from build123d import *

# Parameters (mm, degrees)
SKETCH1_R           = 3.525
SKETCH1_R_2         = 3.53
SKETCH1_R_3         = 3.535
SKETCH1_R_4         = 3.54
SKETCH1_R_5         = 3.545
SKETCH1_R_6         = 3.555
SKETCH1_R_7         = 3.56
SKETCH1_R_8         = 3.565
SKETCH1_R_9         = 3.57
SKETCH1_R_10        = 3.58
SKETCH1_R_11        = 3.585
SKETCH1_R_12        = 3.59
SKETCH1_R_13        = 3.595
SKETCH1_R_14        = 3.605
SKETCH1_R_15        = 3.615
SKETCH1_R_16        = 3.55
SKETCH1_R_17        = 3.575
SKETCH1_R_18        = 3.6
BOSS_EXTRUDE1_DEPTH = 7.62


with BuildPart() as part:
    # Sketch1 → Boss-Extrude1 (new body)
    with BuildSketch(Plane(origin=(0, 0, 0), x_dir=(1, 0, 0), z_dir=(0, 1, 0))):
        Polygon((0, 0), (43.396152207, 0), (43.396152207, 27.288237387), (26.088694952, 27.288237387), (26.088694952, 35.171413764), (0, 35.171413764), align=None)
        with Locations((4.997445859, 4.997445859)):
            Circle(SKETCH1_R, mode=Mode.SUBTRACT)
        with Locations((13.379445859, 4.997445859)):
            Circle(SKETCH1_R_2, mode=Mode.SUBTRACT)
        with Locations((21.761445859, 4.997445859)):
            Circle(SKETCH1_R_3, mode=Mode.SUBTRACT)
        with Locations((30.143445859, 4.997445859)):
            Circle(SKETCH1_R_4, mode=Mode.SUBTRACT)
        with Locations((38.525445859, 4.997445859)):
            Circle(SKETCH1_R_5, mode=Mode.SUBTRACT)
        with Locations((13.379445859, 13.379445859)):
            Circle(SKETCH1_R_6, mode=Mode.SUBTRACT)
        with Locations((21.761445859, 13.379445859)):
            Circle(SKETCH1_R_7, mode=Mode.SUBTRACT)
        with Locations((30.143445859, 13.379445859)):
            Circle(SKETCH1_R_8, mode=Mode.SUBTRACT)
        with Locations((38.525445859, 13.379445859)):
            Circle(SKETCH1_R_9, mode=Mode.SUBTRACT)
        with Locations((13.379445859, 21.761445859)):
            Circle(SKETCH1_R_10, mode=Mode.SUBTRACT)
        with Locations((21.761445859, 21.761445859)):
            Circle(SKETCH1_R_11, mode=Mode.SUBTRACT)
        with Locations((30.143445859, 21.761445859)):
            Circle(SKETCH1_R_12, mode=Mode.SUBTRACT)
        with Locations((38.525445859, 21.761445859)):
            Circle(SKETCH1_R_13, mode=Mode.SUBTRACT)
        with Locations((13.379445859, 30.143445859)):
            Circle(SKETCH1_R_14, mode=Mode.SUBTRACT)
        with Locations((21.761445859, 30.143445859)):
            Circle(SKETCH1_R_15, mode=Mode.SUBTRACT)
        with Locations((4.997445859, 13.379445859)):
            Circle(SKETCH1_R_16, mode=Mode.SUBTRACT)
        with Locations((4.997445859, 21.761445859)):
            Circle(SKETCH1_R_17, mode=Mode.SUBTRACT)
        with Locations((4.997445859, 30.143445859)):
            Circle(SKETCH1_R_18, mode=Mode.SUBTRACT)
    extrude(amount=BOSS_EXTRUDE1_DEPTH)


solid = part.part
Build history of the part. All positions in model axes, mm. A direction names the side the tool comes from. Give positions to 0.01 mm unless a question says otherwise; leave off trailing zeros. Loops run counter-clockwise (first coordinate to the right, second up) from the corner with the lowest first, then second, coordinate; pieces in that order, holes last. Notation, with made-up numbers: (41, -10) -> (46, -10) arc R22 cw to (46, -3) -> close; hole circle Ø6 at (44, 69). An arc over 180 degrees is marked (long way). Answer in a Markdown table with one row per item.
Item 1: Slice it at D-D on x = 39. Write the cut outline in (y, z).
Findings below:
| item | result |
|---|---|
| outline | (0, -27.29) -> (7.62, -27.29) -> (7.62, -25.32) -> (0, -25.32) -> close; (0, -18.2) -> (7.62, -18.2) -> (7.62, -16.92) -> (0, -16.92) -> close; (0, -9.84) -> (7.62, -9.84) -> (7.62, -8.51) -> (0, -8.51) -> close; (0, -1.48) -> (7.62, -1.48) -> (7.62, 0) -> (0, 0) -> close |
Item 2: Probe line 1 along Z through (x, y) = (31.5, 3.75); line 2 along X through (y, z) = (1.75, -14); line 3 along Z through (x, y) = (5.5, 2). List the from-to ranges inside material, lowest first. Write a range as [from, to].
Findings below:
| item | result |
|---|---|
| line 1 | z = [-27.29, -25.09], [-18.44, -16.68], [-10.08, -8.27], [-1.73, 0] |
| line 2 | x = [0, 1.5], [8.49, 9.88], [16.88, 18.26], [25.27, 26.63], [33.65, 35.01], [42.04, 43.4] |
| line 3 | z = [-35.17, -33.71], [-26.58, -25.3], [-18.22, -16.89], [-9.87, -8.49], [-1.51, 0] |
Item 3: Mould opens along X. For faces 3 (the cylindrical face through (18.18, 3.76, -21.92)), 4 (the flat face through (43.396, 4, -13)), 5 (the flat face through (21, 4, 0)) say: pulls with the +X half, pulls with the -X half, needs draft (parallel to the pull), parting line crosses it, or undercut.
Findings below:
| item | result |
|---|---|
| face 3 | undercut |
| face 4 | pulls with the +X half |
| face 5 | needs draft |
Item 4: Slice it at B-B on y = 1.5. Give the number of separate pieces and of enclosed holes in the cut face, plus the area to 3 significant figures.
Findings below:
| item | result |
|---|---|
| separate pieces | 1 |
| enclosed holes | 18 |
| area | 670 mm² |
Item 5: Slice it at A-A on x = 5. Write the cut outline in (y, z), plus the area to 3 significant figures.
Findings below:
| item | result |
|---|---|
| outline | (0, -35.17) -> (7.62, -35.17) -> (7.62, -33.74) -> (0, -33.74) -> close; (0, -26.54) -> (7.62, -26.54) -> (7.62, -25.34) -> (0, -25.34) -> close; (0, -18.19) -> (7.62, -18.19) -> (7.62, -16.93) -> (0, -16.93) -> close; (0, -9.83) -> (7.62, -9.83) -> (7.62, -8.52) -> (0, -8.52) -> close; (0, -1.47) -> (7.62, -1.47) -> (7.62, 0) -> (0, 0) -> close |
| area | 50.8 mm² |
Item 6: Slice it at C-C on z = -4. Write the cut outline in (x, y).
Findings below:
| item | result |
|---|---|
| outline | (0, 0) -> (1.62, 0) -> (1.62, 7.62) -> (0, 7.62) -> close; (8.38, 0) -> (9.99, 0) -> (9.99, 7.62) -> (8.38, 7.62) -> close; (16.77, 0) -> (18.37, 0) -> (18.37, 7.62) -> (16.77, 7.62) -> close; (25.15, 0) -> (26.75, 0) -> (26.75, 7.62) -> (25.15, 7.62) -> close; (33.54, 0) -> (35.12, 0) -> (35.12, 7.62) -> (33.54, 7.62) -> close; (41.93, 0) -> (43.4, 0) -> (43.4, 7.62) -> (41.93, 7.62) -> close |
Item 7: Flat gauge pins, fed straight in: P1, Ø4, axis at y = 2, z = -31.5, coming from the +X side; P2, Ø3, axis at y = 5, z = -4.5, coming from the -X side; P3, Ø4.5, axis at x = 5, z = -30.14, coming from the -Y side; P4, Ø1.5, axis at x = 31.5, y = 1, coming from the -Z side. Where does each tip first touch, or does it go through?
Findings below:
| item | result |
|---|---|
| P1 | stops at x = 26.09 |
| P2 | stops at x = 0 |
| P3 | passes through |
| P4 | stops at z = -27.29 |
Item 8: Tool access for faces 1 (the flat face through (26.089, 4, -31)), 2 (the flat face through (21, 0, -18)): list every direction of +Z, -Z, +X, -X, +Y, -Y with a clear straight run to the whole face (end or side of a thin tool).
Findings below:
| item | result |
|---|---|
| face 1 | -Z, +X, +Y, -Y |
| face 2 | +Z, -Z, +X, -X, -Y |
